```python
from build123d import *

# Parameters (mm, degrees)
SKETCH1_R           = 2.6
BOSS_EXTRUDE1_DEPTH = 3.175
CHAMFER1_SIZE       = 3
SKETCH4_R           = 1.7
CUT_EXTRUDE2_DEPTH  = 4.175
CHAMFER2_SIZE       = 1.5


with BuildPart() as part:
    # Sketch1 → Boss-Extrude1 (new body)
    with BuildSketch(Plane.XY):
        with BuildLine():
            Line((35, -40), (-35, -40))
            ThreePointArc((-35, -40), (-38.535533906, -38.535533906), (-40, -35))
            Line((-40, -35), (-40, 35))
            ThreePointArc((-40, 35), (-38.535533906, 38.535533906), (-35, 40))
            Line((-35, 40), (35, 40))
            ThreePointArc((35, 40), (38.535533906, 38.535533906), (40, 35))
            Line((40, 35), (40, -35))
            ThreePointArc((40, -35), (38.535533906, -38.535533906), (35, -40))
        make_face()
        with Locations((-30, 30)):
            Circle(SKETCH1_R, mode=Mode.SUBTRACT)
        with Locations((30, 30)):
            Circle(SKETCH1_R, mode=Mode.SUBTRACT)
        with Locations((30, -30)):
            Circle(SKETCH1_R, mode=Mode.SUBTRACT)
        with Locations((-30, -30)):
            Circle(SKETCH1_R, mode=Mode.SUBTRACT)
    extrude(amount=BOSS_EXTRUDE1_DEPTH)

    # Chamfer1
    chamfer1_edges = [part.edges().sort_by_distance(p)[0] for p in [
        (-32.6, 30, 0),
        (27.4, 30, 0),
        (27.4, -30, 0),
        (-32.6, -30, 0),
    ]]
    chamfer(chamfer1_edges, length=CHAMFER1_SIZE)

    # Sketch4 → Cut-Extrude2 (cut, through all)
    with BuildSketch(Plane(origin=(0, 0, 0), x_dir=(-1, 0, 0), z_dir=(0, 0, -1))):
        with Locations((-15.5, -20.5)):
            Circle(SKETCH4_R)
        with Locations((-7.75, -7.076606241)):
            Circle(SKETCH4_R)
        with Locations((7.75, -7.076606241)):
            Circle(SKETCH4_R)
        with Locations((15.5, -20.5)):
            Circle(SKETCH4_R)
        with BuildLine():
            Line((9, -17.202559976), (9, -29.202559976))
            ThreePointArc((9, -29.202559976), (8.855473359, -30.808981962), (8.426535201, -32.363810442))
            ThreePointArc((8.426535201, -32.363810442), (9.201851044, -34.807774076), (6.674545917, -35.23997969))
            ThreePointArc((6.674545917, -35.23997969), (0, -38.202559976), (-6.674545917, -35.23997969))
            ThreePointArc((-6.674545917, -35.23997969), (-9.201851044, -34.807774076), (-8.426535201, -32.363810442))
            ThreePointArc((-8.426535201, -32.363810442), (-8.855473359, -30.808981962), (-9, -29.202559976))
            Line((-9, -29.202559976), (-9, -17.202559976))
            ThreePointArc((-9, -17.202559976), (0, -8.202559976), (9, -17.202559976))
        make_face()
    extrude(amount=-CUT_EXTRUDE2_DEPTH, mode=Mode.SUBTRACT)

    # Chamfer2
    chamfer2_edges = [part.edges().sort_by_distance(p)[0] for p in [
        (17.2, -20.5, 0),
        (9.45, -7.076606241, 0),
        (-13.8, -20.5, 0),
        (9.201851044, -34.807774076, 0),
        (-9.201851044, -34.807774076, 0),
        (-6.05, -7.076606241, 0),
    ]]
    chamfer(chamfer2_edges, length=CHAMFER2_SIZE)


solid = part.part
```
Input: part model. Units: mm. Frame: model coordinates. A direction names the side the tool comes from. Round coordinates to 2 decimals unless told otherwise and drop trailing zeros. Loops run counter-clockwise (first coordinate to the right, second up) from the corner with the lowest first, then second, coordinate; pieces in that order, holes last. Notation, with made-up numbers: M -2.75,16.5 L 18.25,16.5 A5 cw 18.25,24.5 Z; hole C 37,46.5 d7. An arc over 180 degrees is marked long. Answer in a Markdown table with one row per item. Add a question column.
1. Section B-B (x = -15.5). Output: boundary loops of the cut face in (y, z) (3 decimals).
2. Set-up query: faces 4 (the face through (0.198, -8.205, 1.565)), 5 (the face through (-30.363, 32.764, 2.812)). Return all of +Z, -Z, +X, -X, +Y, -Y with unobstructed straight access to the full face (end or side cutting, diameter ignored); none if empty.
3. Mould query, pull axis X, two halves, no side actions, for faces 1 (the face through (-17.07, -21.15, 2.33)), 2 (the face through (0, -40, 2)), 3 (the face through (38, 39, 2)). Classes: released by +X, released by -X, zero draft, split by the parting line, or undercut.
4. Contact query for flat-ended pins moving along their axis: pin 1 (6 mm diameter, centred on x = 30, y = -30, fed in from -Z); pin 2 (4 mm diameter, centred on x = 15.5, y = -20.5, fed in from +Z) (3 decimals); pin 3 (2 mm diameter, centred on x = -7.75, y = -33.92, fed in from +Z); pin 4 (8.5 mm diameter, centred on x = -30, y = -30, fed in from -Z). Output: stop coordinate, or through.
5. Section C-C (y = -20.5). Output: boundary loops of the cut face in (x, z) (3 decimals), and give its area (3 significant figures).
6. Section D-D (x = -1). Output: boundary loops of the cut face in (y, z) (3 decimals).
7. Ray query, probe 1 along Y at (x, z) = (30, 3.05); probe 2 along X at (y, z) = (-35, 1.2); probe 3 along Y at (x, z) = (0.5, 1.6). Return the intervals inside material, ascending.
8. Section A-A (y = 30). Output: boundary loops of the cut face in (x, z) (3 decimals), and give its area (3 significant figures).
Values follow:
| question | item | result |
|---|---|---|
| 1 | outline | M -40,0 L -23.7,0 L -22.2,1.5 L -22.2,3.175 L -40,3.175 Z; M -18.8,1.5 L -17.3,0 L 40,0 L 40,3.175 L -18.8,3.175 Z |
| 2 | face 4 | +Z, -Z |
| 2 | face 5 | -Z |
| 3 | face 1 | undercut |
| 3 | face 2 | zero draft |
| 3 | face 3 | released by +X |
| 4 | pin 1 | z = 2.6 |
| 4 | pin 2 | z = 3.175 |
| 4 | pin 3 | through |
| 4 | pin 4 | z = 1.35 |
| 5 | outline | M -40,0 L -18.7,0 L -17.2,1.5 L -17.2,3.175 L -40,3.175 Z; M -13.8,1.5 L -12.3,0 L -9,0 L -9,3.175 L -13.8,3.175 Z; M 9,0 L 12.3,0 L 13.8,1.5 L 13.8,3.175 L 9,3.175 Z; M 17.2,1.5 L 18.7,0 L 40,0 L 40,3.175 L 17.2,3.175 Z |
| 5 | area | 171 mm^2 |
| 6 | outline | M -40,0 L -38.147,0 L -38.147,3.175 L -40,3.175 Z; M -8.258,0 L 40,0 L 40,3.175 L -8.258,3.175 Z |
| 7 | probe 1 | -40 to -32.6, -27.4 to 27.4, 32.6 to 40 |
| 7 | probe 2 | -40 to -9.44, 9.44 to 40 |
| 7 | probe 3 | -40 to -38.19, -8.22 to 40 |
| 8 | outline | M -40,0 L -35.6,0 L -32.6,3 L -32.6,3.175 L -40,3.175 Z; M -27.4,3 L -24.4,0 L 24.4,0 L 27.4,3 L 27.4,3.175 L -27.4,3.175 Z; M 32.6,3 L 35.6,0 L 40,0 L 40,3.175 L 32.6,3.175 Z |
| 8 | area | 203 mm^2 |
